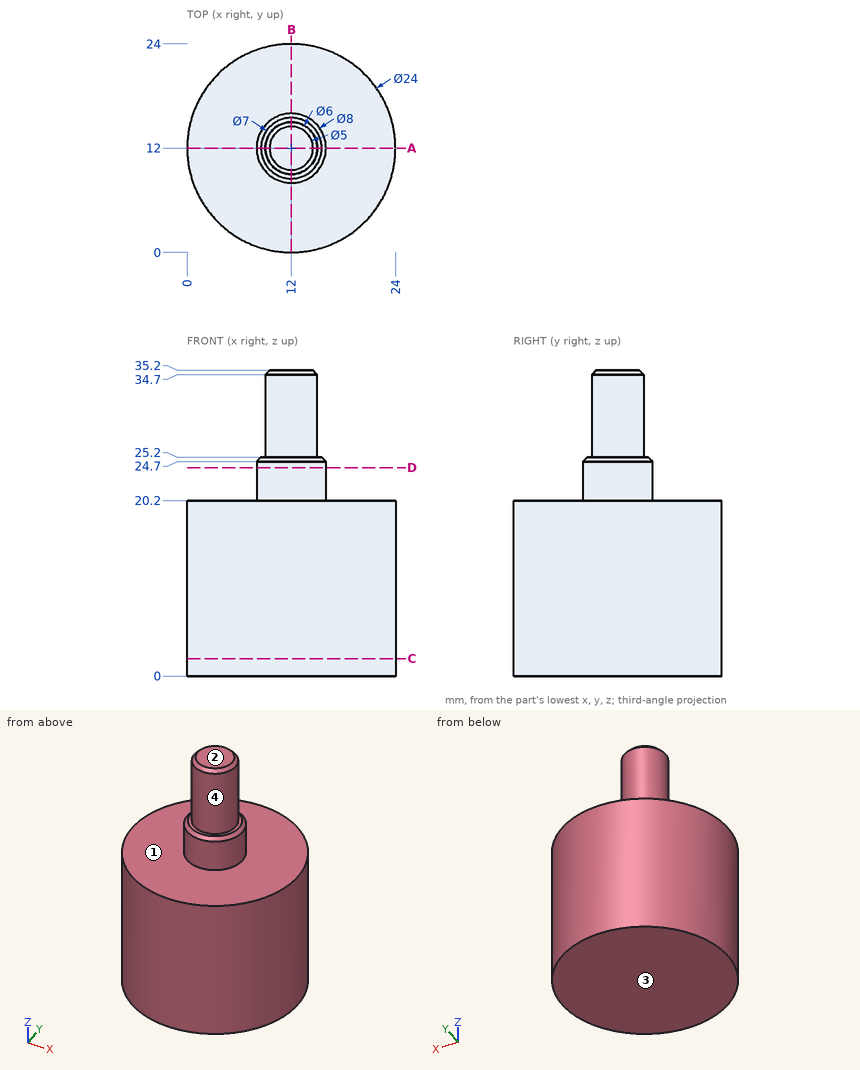
Could you check a few things on this drawing? It's one solid part, dimensions in mm from its lowest x, y, z. A direction names the side the tool comes from. Give positions to 0.01 mm unless a question says otherwise; leave off trailing zeros. Order: outer loops, then holes, each group sorted by start corner. A loop starts at its lowest first (then second) coordinate and runs counter-clockwise, first axis right, second up. Notation, with made-up numbers: M 89.5,25 L 137.5,25 A10 cw 137.5,41 Z; hole C 4.5,19.25 d9. An arc over 180 degrees is marked long. Use one line per item in the form item = value.
Item 1: If we section it at D-D, the plane z = 24: Write out the boundary of the cut face in (x, y).
Values follow:
outline = C 12,12 d8
Item 2: If we section it at C-C, the plane z = 2: Write out the boundary of the cut face in (x, y).
Values follow:
outline = C 12,12 d24
Item 3: If I drill on line 1 along Z through (x, y) = (18.5, 5); line 2 along Z through (x, y) = (10.5, 15.25); line 3 along Y through (x, z) = (9.25, 29), over which ranges is the centre line in solid material (lowest first)? Write a range as [from, to].
Values follow:
line_1 = [0, 20.2]
line_2 = [0, 25.12]
line_3 = [10.8, 13.2]
Item 4: Thinking about a two-plate mould opening in X: for the marked faces 3 and 4, which applies, pulls with the +X half, pulls with the -X half, needs draft (parallel to the pull), parting line crosses it, or undercut?
Values follow:
face_3 = needs draft
face_4 = parting line crosses it
Item 5: If we section it at A-A, the plane y = 12: Write out the boundary of the cut face in (x, z), and give its area (3 significant figures).
Values follow:
outline = M 0,0 L 24,0 L 24,20.2 L 16,20.2 L 16,24.7 L 15.5,25.2 L 15,25.2 L 15,34.7 L 14.5,35.2 L 9.5,35.2 L 9,34.7 L 9,25.2 L 8.5,25.2 L 8,24.7 L 8,20.2 L 0,20.2 Z
area = 584 mm^2
Item 6: For the marked faces 1 and 2, which set-ups out of +Z, -Z, +X, -X, +Y, -Y let a thin tool reach every point of the face, with its end or its side?
Values follow:
face_1 = +Z
face_2 = +Z, +X, -X, +Y, -Y
Item 7: Will these pins go through, and if not, where does the flat tip stop? pin 1 Ø12 at (x, y) = (7.5, 8.5) entering from +Z; pin 2 Ø1.5 at (x, y) = (17, 10.5) entering from +Z; pin 3 Ø4 at (y, z) = (10, 25.5) entering from -X; pin 4 Ø8 at (x, z) = (18, 8) entering from +Y.
Values follow:
pin_1 = 35.2
pin_2 = 20.2
pin_3 = 8
pin_4 = 23.83
